Design review of the part built by this model. Coordinates are the model's own, in mm. Face numbers are marked on the shaded views. Give positions to 0.01 mm unless a question says otherwise; leave off trailing zeros. Loops run counter-clockwise (first coordinate to the right, second up) from the corner with the lowest first, then second, coordinate; pieces in that order, holes last. Notation, with made-up numbers: (21.5, 9) -> (78.5, 9) arc R23 ccw to (78.5, 36) -> close; hole circle Ø2 at (12, 46). An arc over 180 degrees is marked (long way). Answer in a Markdown table with one row per item. Add a question column.
(1) Consider section B-B on z = 0. Write out the cut boundary in (x, y), then the cut area to 3 significant figures.
(2) Consider section C-C on y = 18. Write out the cut boundary in (x, z), then the cut area to 3 significant figures.
(3) Consider section A-A on x = 0. Write out the cut boundary in (y, z).
(4) Draft analysis for pull direction Z (two halves, no side actions). For the marked faces 1, 2 and 3, state which applies: +Z half, -Z half, draft (parallel to the pull), parting line (faces both ways), or undercut.
(5) For line 1 (X direction, y = 12, z = 0); line 2 (X direction, y = 21, z = -5); line 3 (Z direction, x = -3.5, y = 16.5), list the stretches that pass through material, from the lowest coordinate up.
(6) For pin 1 (4 mm diameter, centred on y = 16.5, z = 3, fed in from -X); pin 2 (4 mm diameter, centred on x = -19, y = 27, fed in from -Z); pin 3 (1 mm diameter, centred on x = -21.5, y = 41, fed in from -Z), all flat-tipped, find the tip position at first contact; note any pin that passes through.
from build123d import *
from OCP.BRepFilletAPI import BRepFilletAPI_MakeChamfer

# Parameters (mm, degrees)
SKETCH1_R           = 35
BOSS_EXTRUDE1_DEPTH = 45.475969
SKETCH2_R           = 20.508937662
CUT_EXTRUDE1_DEPTH  = 68.216543771
CHAMFER1_SIZE       = 1.535786
CHAMFER1_SIZE2      = 0.886687


with BuildPart() as part:
    # Sketch1 → Boss-Extrude1 (new body)
    with BuildSketch(Plane(origin=(0, 0, 0), x_dir=(1, 0, 0), z_dir=(0, 1, 0))):
        with Locations(Location((0, 0, 0), (0, 0, 270))):
            Circle(SKETCH1_R)
    extrude(amount=BOSS_EXTRUDE1_DEPTH)

    # Sketch2 → Cut-Extrude1 (cut, through all)
    with BuildSketch(Plane(origin=(0, 0, 0), x_dir=(1, 0, 0), z_dir=(0, 1, 0))):
        with Locations(Location((0, 0, 0), (0, 0, 270))):
            Circle(SKETCH2_R)
    extrude(amount=CUT_EXTRUDE1_DEPTH, mode=Mode.SUBTRACT)

    # Chamfer1: one chamfer whose edges measure the first distance from different faces: ONE call of the kernel's chamfer builder (chamfer() names one face for all edges)
    chamfer1_edges_1 = [part.edges().sort_by_distance(p)[0] for p in [
        (0, 0, -35),
    ]]
    chamfer1_side_1 = [part.faces().sort_by_distance(p)[0] for p in [
        (0, 22.7379845, -35),
    ]]
    chamfer1_edges_2 = [part.edges().sort_by_distance(p)[0] for p in [
        (0, 45.475969, -35),
    ]]
    chamfer1_side_2 = [part.faces().sort_by_distance(p)[0] for p in [
        (0, 45.475969, -34.010050506),
    ]]
    chamfer1_edges_3 = [part.edges().sort_by_distance(p)[0] for p in [
        (0, 0, -20.508937662),
    ]]
    chamfer1_side_3 = [part.faces().sort_by_distance(p)[0] for p in [
        (0, 0, -34.010050506),
    ]]
    chamfer1_edges_4 = [part.edges().sort_by_distance(p)[0] for p in [
        (0, 45.475969, -20.508937662),
    ]]
    chamfer1_side_4 = [part.faces().sort_by_distance(p)[0] for p in [
        (0, 22.7379845, -20.508937662),
    ]]
    chamfer1 = BRepFilletAPI_MakeChamfer(part.part.solid().wrapped)
    for e in chamfer1_edges_1:
        chamfer1.Add(CHAMFER1_SIZE, CHAMFER1_SIZE2, e.wrapped, chamfer1_side_1[0].wrapped)  # the first distance lies on this face
    for e in chamfer1_edges_2:
        chamfer1.Add(CHAMFER1_SIZE, CHAMFER1_SIZE2, e.wrapped, chamfer1_side_2[0].wrapped)  # the first distance lies on this face
    for e in chamfer1_edges_3:
        chamfer1.Add(CHAMFER1_SIZE, CHAMFER1_SIZE2, e.wrapped, chamfer1_side_3[0].wrapped)  # the first distance lies on this face
    for e in chamfer1_edges_4:
        chamfer1.Add(CHAMFER1_SIZE, CHAMFER1_SIZE2, e.wrapped, chamfer1_side_4[0].wrapped)  # the first distance lies on this face
    add(Compound.cast(chamfer1.Shape()), mode=Mode.REPLACE)


solid = part.part
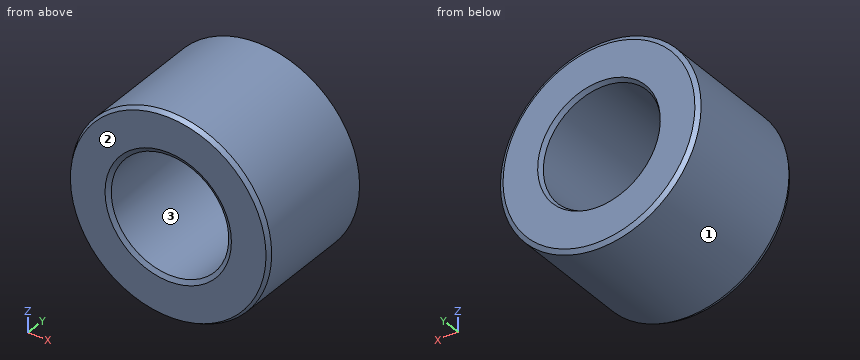
Values follow:
| question | item | result |
|---|---|---|
| 1 | outline | (-35, 1.54) -> (-34.11, 0) -> (-22.04, 0) -> (-20.51, 0.89) -> (-20.51, 43.94) -> (-21.4, 45.48) -> (-33.46, 45.48) -> (-35, 44.59) -> close; (20.51, 0.89) -> (22.04, 0) -> (34.11, 0) -> (35, 1.54) -> (35, 44.59) -> (33.46, 45.48) -> (21.4, 45.48) -> (20.51, 43.94) -> close |
| 1 | area | 1,310 mm2 |
| 2 | outline | circle Ø70 at (0, 0); hole circle Ø41.02 at (0, 0) |
| 2 | area | 2,530 mm2 |
| 3 | outline | (0, -34.11) -> (1.54, -35) -> (44.59, -35) -> (45.48, -33.46) -> (45.48, -21.4) -> (43.94, -20.51) -> (0.89, -20.51) -> (0, -22.04) -> close; (0, 22.04) -> (0.89, 20.51) -> (43.94, 20.51) -> (45.48, 21.4) -> (45.48, 33.46) -> (44.59, 35) -> (1.54, 35) -> (0, 34.11) -> close |
| 4 | face 1 | parting line |
| 4 | face 2 | draft |
| 4 | face 3 | undercut |
| 5 | line 1 | -35 to -20.51, 20.51 to 35 |
| 5 | line 2 | -34.64 to -19.89, 19.89 to 34.64 |
| 5 | line 3 | -34.82 to -20.21, 20.21 to 34.82 |
| 6 | pin 1 | x = -34.99 |
| 6 | pin 2 | z = -30.59 |
| 6 | pin 3 | z = -28 |
